```python
from build123d import *

# Parameters (mm, degrees)
F0_W      = 147
F0_H      = 45.5
F0_W_2    = 67
F0_H_2    = 3.3
F0_R      = 3.5
F0_W_3    = 72.2
F0_H_3    = 24.3
F1_DEPTH  = 1.5
F2_DEPTH  = 1.5
F3_DEPTH  = 1.5
F4_DEPTH  = 1.5
F5_DEPTH  = 1.5
F6_R      = 2.5
F7_DEPTH  = 3
F8_R      = 1.75
F9_DEPTH  = 6
F10_R     = 2.5
F11_DEPTH = 3
F12_R     = 1.75
F13_DEPTH = 25
F14_R     = 2.5
F15_DEPTH = 3
F16_R     = 1.75
F17_DEPTH = 25
F18_R     = 2.5
F19_DEPTH = 3
F20_R     = 1.75
F21_DEPTH = 25


with BuildPart() as f1:
    # F0 (on Top) → F1 (new body)
    with BuildSketch(Plane.XY):
        Rectangle(F0_W, F0_H)
        with Locations((-4.4, -15.3125505805)):
            Rectangle(F0_W_2, F0_H_2, mode=Mode.SUBTRACT)
        with BuildLine():
            ThreePointArc((53.7276520505, -15.79), (56.5004484729, -6.85), (59.2732448953, -15.79))
            Line((59.2732448953, -15.79), (53.7276520505, -15.79))
        make_face(mode=Mode.SUBTRACT)
        with Locations((-57, 0)):
            Circle(F0_R, mode=Mode.SUBTRACT)
        with Locations((-4.4, 0)):
            Rectangle(F0_W_3, F0_H_3, mode=Mode.SUBTRACT)
        with BuildLine():
            ThreePointArc((53.7272035776, 7.71), (56.5, 16.65), (59.2727964224, 7.71))
            Line((59.2727964224, 7.71), (53.7272035776, 7.71))
        make_face(mode=Mode.SUBTRACT)
    extrude(amount=F1_DEPTH)

    # F0 (on Top) → F2 (join)
    with BuildSketch(Plane.XY):
        Rectangle(F0_W, F0_H)
        with Locations((-4.4, -15.3125505805)):
            Rectangle(F0_W_2, F0_H_2, mode=Mode.SUBTRACT)
        with BuildLine():
            ThreePointArc((53.7276520505, -15.79), (56.5004484729, -6.85), (59.2732448953, -15.79))
            Line((59.2732448953, -15.79), (53.7276520505, -15.79))
        make_face(mode=Mode.SUBTRACT)
        with Locations((-57, 0)):
            Circle(F0_R, mode=Mode.SUBTRACT)
        with Locations((-4.4, 0)):
            Rectangle(F0_W_3, F0_H_3, mode=Mode.SUBTRACT)
        with BuildLine():
            ThreePointArc((53.7272035776, 7.71), (56.5, 16.65), (59.2727964224, 7.71))
            Line((59.2727964224, 7.71), (53.7272035776, 7.71))
        make_face(mode=Mode.SUBTRACT)
    extrude(amount=F2_DEPTH)

    # F0 (on Top) → F3 (join)
    with BuildSketch(Plane.XY):
        Rectangle(F0_W, F0_H)
        with Locations((-4.4, -15.3125505805)):
            Rectangle(F0_W_2, F0_H_2, mode=Mode.SUBTRACT)
        with BuildLine():
            ThreePointArc((53.7276520505, -15.79), (56.5004484729, -6.85), (59.2732448953, -15.79))
            Line((59.2732448953, -15.79), (53.7276520505, -15.79))
        make_face(mode=Mode.SUBTRACT)
        with Locations((-57, 0)):
            Circle(F0_R, mode=Mode.SUBTRACT)
        with Locations((-4.4, 0)):
            Rectangle(F0_W_3, F0_H_3, mode=Mode.SUBTRACT)
        with BuildLine():
            ThreePointArc((53.7272035776, 7.71), (56.5, 16.65), (59.2727964224, 7.71))
            Line((59.2727964224, 7.71), (53.7272035776, 7.71))
        make_face(mode=Mode.SUBTRACT)
    extrude(amount=F3_DEPTH)

    # F0 (on Top) → F4 (join, symmetric)
    with BuildSketch(Plane.XY):
        with Locations((-4.4, -15.3125505805)):
            Rectangle(F0_W_2, F0_H_2)
    extrude(amount=F4_DEPTH, both=True)

    # F5 (add): a face of the model
    f5_faces = [f1.faces().sort_by_distance(p)[0] for p in [
        (-4.4, -15.3125505805, -1.5),
    ]]
    extrude(f5_faces, amount=F5_DEPTH)

    # F6 (on face) → F7 (join)
    with BuildSketch(Plane.XY):
        with Locations((33.1043936312, 16.1594673991)):
            Circle(F6_R)
    extrude(amount=-F7_DEPTH)

    # F8 (on face) → F9 (cut)
    with BuildSketch(Plane(origin=(0, 0, -3), x_dir=(1, 0, 0), z_dir=(0, 0, -1))):
        with Locations((33.1043936312, -16.1594673991)):
            Circle(F8_R)
    extrude(amount=-F9_DEPTH, mode=Mode.SUBTRACT)

    # F10 (on face) → F11 (join)
    with BuildSketch(Plane.XY):
        with Locations((-41.8984927237, 16.1572918296)):
            Circle(F10_R)
    extrude(amount=-F11_DEPTH)

    # F12 (on face) → F13 (cut)
    with BuildSketch(Plane(origin=(0, 0, -3), x_dir=(1, 0, 0), z_dir=(0, 0, -1))):
        with Locations((-41.8984927237, -16.1572918296)):
            Circle(F12_R)
    extrude(amount=-F13_DEPTH, mode=Mode.SUBTRACT)

    # F14 (on face) → F15 (join)
    with BuildSketch(Plane.XY):
        with Locations((-41.893761605, -14.8712657392)):
            Circle(F14_R)
    extrude(amount=-F15_DEPTH)

    # F16 (on face) → F17 (cut)
    with BuildSketch(Plane(origin=(0, 0, -3), x_dir=(1, 0, 0), z_dir=(0, 0, -1))):
        with Locations((-41.893761605, 14.8712657392)):
            Circle(F16_R)
    extrude(amount=-F17_DEPTH, mode=Mode.SUBTRACT)

    # F18 (on face) → F19 (join)
    with BuildSketch(Plane.XY):
        with Locations((33.1018306315, -14.8555124179)):
            Circle(F18_R)
    extrude(amount=-F19_DEPTH)

    # F20 (on face) → F21 (cut)
    with BuildSketch(Plane(origin=(0, 0, -3), x_dir=(1, 0, 0), z_dir=(0, 0, -1))):
        with Locations((33.1018306315, 14.8555124179)):
            Circle(F20_R)
    extrude(amount=-F21_DEPTH, mode=Mode.SUBTRACT)


solid = f1.part
```
Work out the finished part from the listing and answer in its coordinate system (mm). A direction names the side the tool comes from. Give positions to 0.01 mm unless a question says otherwise; leave off trailing zeros. Order: outer loops, then holes, each group sorted by start corner. A loop starts at its lowest first (then second) coordinate and runs counter-clockwise, first axis right, second up. Notation, with made-up numbers: (13, 23.25) - (53, 23.25) arc R12 cw to (53, 31.25) - close; hole circle Ø11 at (80.25, 81.25). An arc over 180 degrees is marked (long way). One line per item, written item: value. Start each with the question number.
1. Section D-D, the plane x = 56.5 is taken. Write down the section's boundary in (y, z), then the cut area to 3 significant figures.
2. Section B-B, the plane z = -2.3 is taken. Count the separate pieces of the cut face and the enclosed holes in it, then the cut area to 3 significant figures.
3. Which of the six approach directions +Z, -Z, +X, -X, +Y, -Y give full straight-line access (tool end or side, diameter ignored) to faces 1 (the face through (-44.396, 16.267, -1.479)), 2 (the face through (-37.9, -15, -1)), 3 (the face through (31, -15, -3)), 4 (the face through (-5, -16.963, -1))?
4. Consider line 1 (X direction, y = -11.75, z = 0.4); line 2 (Y direction, x = -16, z = 0.85); line 3 (X direction, y = 6, z = 0.6). Determine where each line is inside the solid, lowest interval first.
5. Section C-C, the plane x = -25 is taken. Write down the section's boundary in (y, z), then the cut area to 3 significant figures.
6. Section A-A, the plane y = 0 is taken. Write down the section's boundary in (x, z), then the cut area to 3 significant figures.
7. Each of these flat-tipped pins is pushed along its axis until it touches: pin 1 Ø4.5 at (x, y) = (33.1, 16.16) entering from -Z; pin 2 Ø0.9 at (x, z) = (7.5, -1) entering from -Y; pin 3 Ø1.5 at (y, z) = (-10, -1) entering from -X; pin 4 Ø12.5 at (x, y) = (56.5, 11.75) entering from -Z. Where does it stop, or does it pass through?
8. For a pull along Y with two mould halves and no side action, classify faces 5 (the face through (-5, -13.663, -1)), 6 (the face through (29.1, -15, -1)), 7 (the face through (30.607, 16.269, -1.479)) as released by +Y, released by -Y, zero draft, split by the parting line, or undercut.
Filled sheet:
1. outline: (-22.75, 0) - (-15.79, 0) - (-15.79, 1.5) - (-22.75, 1.5) - close; (-6.85, 0) - (7.71, 0) - (7.71, 1.5) - (-6.85, 1.5) - close; (16.65, 0) - (22.75, 0) - (22.75, 1.5) - (16.65, 1.5) - close
1. area: 41.4 mm²
2. separate pieces: 5
2. enclosed holes: 4
2. area: 261 mm²
3. face 1: -Z
3. face 2: -Z, +Y, -Y
3. face 3: -Z, +X, -X, +Y, -Y
3. face 4: -Z, -Y
4. line 1: -73.5 to -40.5, 31.7 to 51.6, 61.4 to 73.5
4. line 2: -22.75 to -12.15, 12.15 to 22.75
4. line 3: -73.5 to -40.5, 31.7 to 73.5
5. outline: (-22.75, 0) - (-16.96, 0) - (-16.96, -3) - (-13.66, -3) - (-13.66, 0) - (-12.15, 0) - (-12.15, 1.5) - (-22.75, 1.5) - close; (12.15, 0) - (22.75, 0) - (22.75, 1.5) - (12.15, 1.5) - close
5. area: 41.7 mm²
6. outline: (-73.5, 0) - (-60.5, 0) - (-60.5, 1.5) - (-73.5, 1.5) - close; (-53.5, 0) - (-40.5, 0) - (-40.5, 1.5) - (-53.5, 1.5) - close; (31.7, 0) - (73.5, 0) - (73.5, 1.5) - (31.7, 1.5) - close
6. area: 102 mm²
7. pin 1: z = -3
7. pin 2: y = -16.96
7. pin 3: through
7. pin 4: z = 0
8. face 5: released by +Y
8. face 6: zero draft
8. face 7: undercut
